from build123d import *

# Parameters (mm, degrees)
BOSS_EXTRUDE2_DEPTH                                 = 5
CSK_FOR_M3_COUNTERSUNK_FLAT_HEAD_SCREW1_D           = 3.4
CSK_FOR_M3_COUNTERSUNK_FLAT_HEAD_SCREW1_DEPTH       = 5
CSK_FOR_M3_COUNTERSUNK_FLAT_HEAD_SCREW1_CSINK_D     = 6.3
CSK_FOR_M3_COUNTERSUNK_FLAT_HEAD_SCREW1_CSINK_ANGLE = 90
CSK_FOR_M3_COUNTERSUNK_FLAT_HEAD_SCREW1_TIP         = 1.021463052
CUT_EXTRUDE1_REACH                                  = 103.946
SKETCH4_W                                           = 18
SKETCH4_H                                           = 60
SKETCH5_R                                           = 25
CUT_EXTRUDE2_DEPTH                                  = 1
FILLET1_R                                           = 10


with BuildPart() as part:
    # Sketch1 → Boss-Extrude2 (new body)
    with BuildSketch(Plane.XY):
        with BuildLine():
            Line((-23.664319132, 68), (23.664319132, 68))
            ThreePointArc((23.664319132, 68), (0, -72), (-23.664319132, 68))
        make_face()
    extrude(amount=BOSS_EXTRUDE2_DEPTH)

    # Chamfer1: read off the stored shape, not the designer's step
    # Chamfer1 outline → Chamfer1 (revolve, cut)
    with BuildSketch(Plane.XZ):
        Polygon((72.000000172, 5.000000172), (67, 0), (72.000000172, 0), align=None)
    revolve(axis=Axis((0, 0, 0), (0, 0, 1)), mode=Mode.SUBTRACT)

    # CSK for M3 Countersunk Flat Head Screw1
    with Locations(Plane.XY.offset(5)):
        with Locations((15, -38.31), (-15, -38.31), (0, -52.31)):
            CounterSinkHole(CSK_FOR_M3_COUNTERSUNK_FLAT_HEAD_SCREW1_D / 2, CSK_FOR_M3_COUNTERSUNK_FLAT_HEAD_SCREW1_CSINK_D / 2, depth=CSK_FOR_M3_COUNTERSUNK_FLAT_HEAD_SCREW1_DEPTH, counter_sink_angle=CSK_FOR_M3_COUNTERSUNK_FLAT_HEAD_SCREW1_CSINK_ANGLE)
            with Locations((0, 0, -(CSK_FOR_M3_COUNTERSUNK_FLAT_HEAD_SCREW1_DEPTH + CSK_FOR_M3_COUNTERSUNK_FLAT_HEAD_SCREW1_TIP / 2))):  # 118° drill point
                Cone(0, CSK_FOR_M3_COUNTERSUNK_FLAT_HEAD_SCREW1_D / 2, CSK_FOR_M3_COUNTERSUNK_FLAT_HEAD_SCREW1_TIP, mode=Mode.SUBTRACT)

    # Cut-Extrude1: up to this face of the body (flat: up to its plane)
    cut_extrude1_end = Plane(part.part.faces().sort_by_distance((0, 0.083165236, 0))[0])
    # Sketch4 → Cut-Extrude1 (cut, up to the picked face)
    with BuildSketch(Plane.XY.offset(5), mode=Mode.PRIVATE) as cut_extrude1_sk1:
        with Locations((-1.5, 38)):
            Rectangle(SKETCH4_W, SKETCH4_H)
    cut_extrude1_tool1 = split(extrude(cut_extrude1_sk1.sketch, amount=-CUT_EXTRUDE1_REACH, mode=Mode.PRIVATE), bisect_by=cut_extrude1_end, keep=Keep.BOTH, mode=Mode.PRIVATE)
    add(cut_extrude1_tool1.solids().sort_by(Axis((-1.5, 38, 5), (0, 0, -1)))[0], mode=Mode.SUBTRACT)

    # Sketch5 → Cut-Extrude2 (cut)
    with BuildSketch(Plane.XY.offset(5)):
        with Locations((0, 61.9)):
            Circle(SKETCH5_R)
    extrude(amount=-CUT_EXTRUDE2_DEPTH, mode=Mode.SUBTRACT)

    # Fillet1
    # the kernel refuses this fillet: 10 mm, written as the material it adds along each edge
    with BuildSketch(Plane(origin=(-10.5, 8, 5), x_dir=(1, 0, 0), z_dir=(0, 0, -1)), Plane(origin=(7.5, 8, 5), x_dir=(0, 1, 0), z_dir=(0, 0, -1))) as fillet1_piece_1:
        with BuildLine():
            CenterArc((FILLET1_R, -FILLET1_R), FILLET1_R, 90, 90)
            Line((0, -FILLET1_R), (0, 0))
            Line((0, 0), (FILLET1_R, 0))
        make_face()
    extrude(amount=5)


solid = part.part
Build history of the part. All positions in model axes, mm. A direction names the side the tool comes from. Give positions to 0.01 mm unless a question says otherwise; leave off trailing zeros. Use one line per item in the form item = value. Start each with the question number.
1. Probe line 1 (X direction, y = -39, z = 0.3); line 2 (X direction, y = -38.31, z = 2.3); line 3 (Y direction, x = 15, z = 2.4). List the from-to ranges inside material, lowest first. Write a range as [from, to].
2. Drop flat-ended pins along their axis: pin 1 Ø3 at (x, y) = (15, -38.31) entering from +Z; pin 2 Ø2 at (y, z) = (17.5, 1) entering from +X; pin 3 Ø9 at (x, y) = (19.5, 50.5) entering from +Z; pin 4 Ø1.5 at (y, z) = (-56, 2.5) entering from +X. Give the stop position or say it passes through.
3. 3-axis set-ups, long thin cutter, end or side, ignore diameter. For faces 1 (the face through (21.634, 49.371, 4.507)), 2 (the face through (-10.5, 43, 3)), 3 (the face through (1, -3, 5)): which of +Z, -Z, +X, -X, +Y, -Y reach the whole face in a straight line?
4. Band-saw the part on A-A on y = -38.31. Count the separate pieces of the cut face and the enclosed holes in it, plus the area to 3 significant figures.
Conclusion:
q1.line_1 = [-54.85, -16.55], [-13.45, 13.45], [16.55, 54.85]
q1.line_2 = [-57.75, -16.7], [-13.3, 13.3], [16.7, 57.75]
q1.line_3 = [-67.76, -40.01], [-36.61, 67.76]
q2.pin_1 = through
q2.pin_2 = 66.78
q2.pin_3 = 5
q2.pin_4 = 42.76
q3.face_1 = +Z
q3.face_2 = +Z, -Z, +Y
q3.face_3 = +Z, +X, -X, +Y, -Y
q4.separate_pieces = 3
q4.enclosed_holes = 0
q4.area = 542 mm²
